Work out the finished part from the listing and answer in its coordinate system (mm). A direction names the side the tool comes from. Give positions to 0.01 mm unless a question says otherwise; leave off trailing zeros. Order: outer loops, then holes, each group sorted by start corner. A loop starts at its lowest first (then second) coordinate and runs counter-clockwise, first axis right, second up. Notation, with made-up numbers: (44, 56.5) - (87, 56.5) arc R26 ccw to (87, 91.5) - close; hole circle Ø8 at (71.5, 17). An arc over 180 degrees is marked (long way). Put each result on its own line as item: value.
Autodesk Fusion 360 part; units mm, degrees
sphere "SpherePrimitive1" add diameter 38 placed x (1, 0, 0) y (0, 0, -1) z (0, 1, 0) at (0, 0, 0)
sketch "Sketch2" plane through (0, 0, 0) normal (1, 0, 0) x (0, 0, -1)
  circle A0 centre (0, 0) radius 1.5
  dimension "d2" = 3
sketch "Sketch3" plane through (0, 0, 0) normal (0, 0, 1) x (1, 0, 0)
  circle A0 centre (0, 0) radius 1.5
  dimension "d3" = 3
sketch "Sketch4" plane through (0, 0, 0) normal (0, 1, 0) x (1, 0, 0)
  circle A0 centre (0, 0) radius 4.5
  dimension "d4" = 9
extrude "Extrude1" cut sketch "Sketch4" along normal blind 50
extrude "Extrude2" cut sketch "Sketch2" along normal mid plane 100
extrude "Extrude3" cut sketch "Sketch3" along normal mid plane 120
(1) Section B-B, the plane x = 8 is taken. Write down the section's boundary in (y, z).
Geometry check:
outline: circle Ø34.47 at (0, 0); hole circle Ø3 at (0, 0)
(2) Section D-D, the plane x = -2.5 is taken. Write down the section's boundary in (y, z).
Geometry check:
outline: (0, -3.74) - (0, -1.5) arc R1.5 cw to (0, 1.5) - (0, 3.74) - (18.46, 3.74) arc R18.83 ccw (long way) to (18.46, -3.74) - close
(3) Straight lines are drawn through the part: line 1 (Z direction, x = 2, y = 15); line 2 (Z direction, x = 5, y = -1); line 3 (X direction, y = 0, z = -5). For each, find the intervals that lie inside material, in ascending order.
Geometry check:
line 1: z = -11.49 to -4.03, 4.03 to 11.49
line 2: z = -18.3 to -1.12, 1.12 to 18.3
line 3: x = -18.33 to -1.5, 1.5 to 18.33
(4) Determine the mould class of faces 1 (the face through (11.442, -1.487, 0.195)), 2 (the face through (-0.325, -1.464, -11.442)) for opening direction X: pulls with the +X half, pulls with the -X half, needs draft (parallel to the pull), parting line crosses it, or undercut.
Geometry check:
face 1: needs draft
face 2: undercut
(5) Section C-C, the plane y = -9.5 is taken. Write down the section's boundary in (x, z).
Geometry check:
outline: circle Ø32.91 at (0, 0)
(6) Section A-A, the plane z = 17 is taken. Write down the section's boundary in (x, y), then the cut area to 3 significant figures.
Geometry check:
outline: circle Ø16.97 at (0, 0); hole circle Ø3 at (0, 0)
area: 219 mm²
(7) A tool of negligible diameter and unlimited length cuts with its end or side. For faces 3 (the face through (-0.195, -1.487, 11.442)), 4 (the face through (3, 0, 3)), from which of +Z, -Z, +X, -X, +Y, -Y can it reach the whole face along a straight path? Write none if from no direction.
Geometry check:
face 3: +Z, -Z
face 4: +Y
(8) Given pin 1 (8 mm diameter, centred on x = 13, y = 11.5, fed in from -Z); pin 2 (1.4 mm diameter, centred on x = 2.5, z = -2.5, fed in from +Y); pin 3 (1.5 mm diameter, centred on x = 10, y = -5.5, fed in from -Z), each flat-ended and moving along its own axis, determine where each tip first touches the part or whether it passes through.
Geometry check:
pin 1: stops at z = -13.51
pin 2: stops at y = 0
pin 3: stops at z = -15.73
